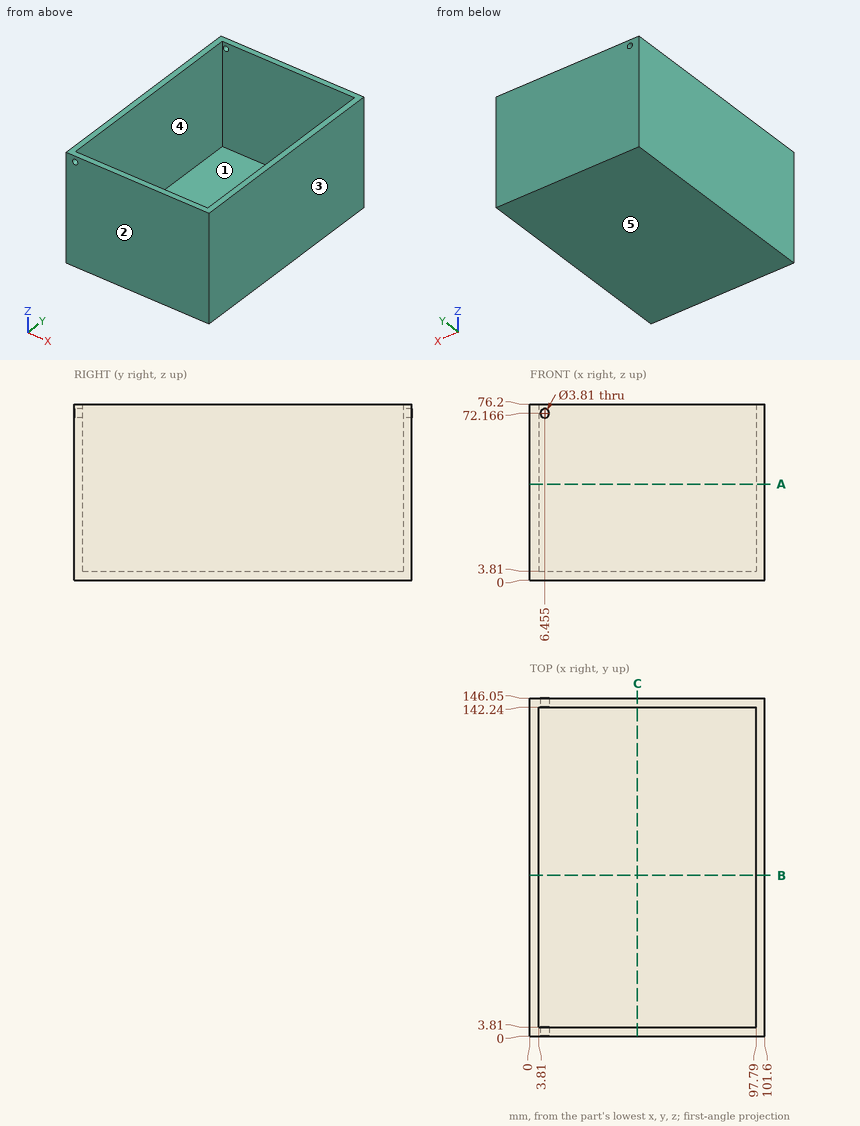
Can you work these out from the drawing? Everything is in mm from the part's minimum corner. A direction names the side the tool comes from. Round coordinates to 2 decimals unless told otherwise and drop trailing zeros. Order: outer loops, then holes, each group sorted by start corner. A loop starts at its lowest first (then second) coordinate and runs counter-clockwise, first axis right, second up. Notation, with made-up numbers: (42, -18) -> (50, -18) arc R12 ccw to (50, 0) -> close; hole circle Ø1 at (33, -28). An arc over 180 degrees is marked (long way). Return JSON: item names as keys, results as strings. Group by question number.
1. We'd pull the mould along Y, two halves only. Please class the marked faces 1, 2 and 3: released by +Y, released by -Y, zero draft, split by the parting line, or undercut.
2. I need wall thicknesses on line 1 (Y direction, x = 49.5, z = 57.5); line 2 (X direction, y = 119, z = 46.5); line 3 (Z direction, x = 14.5, y = 133). Which ranges of each line are inside material? Lowest first, please. Write a range as [from, to].
3. If we section it at C-C, the plane x = 46.5: Write out the boundary of the cut face in (y, z).
4. Will these pins go through, and if not, where does the flat tip stop? pin 1 (10 mm diameter, centred on x = 47.5, y = 106, fed in from +Z); pin 2 (3 mm diameter, centred on x = 6.46, z = 72.17, fed in from +Y).
5. Which directions (+Z, -Z, +X, -X, +Y, -Y) give clear straight access to the entire face, cutting with the end or side of a thin tool? Please do the marked faces 4 and 5.
6. If we section it at B-B, the plane y = 69.5: Write out the boundary of the cut face in (x, z).
7. If we section it at A-A, the plane z = 41.5: Write out the boundary of the cut face in (x, y).
Output values:
{
 "1": {"face 1": "undercut", "face 2": "released by -Y", "face 3": "zero draft"},
 "2": {"line 1": "[0, 3.81], [142.24, 146.05]", "line 2": "[0, 3.81], [97.79, 101.6]", "line 3": "[0, 3.81]"},
 "3": {"outline": "(0, 0) -> (146.05, 0) -> (146.05, 76.2) -> (142.24, 76.2) -> (142.24, 3.81) -> (3.81, 3.81) -> (3.81, 76.2) -> (0, 76.2) -> close"},
 "4": {"pin 1": "z = 3.81", "pin 2": "through"},
 "5": {"face 4": "+Z", "face 5": "-Z, +X, -X, +Y, -Y"},
 "6": {"outline": "(0, 0) -> (101.6, 0) -> (101.6, 76.2) -> (97.79, 76.2) -> (97.79, 3.81) -> (3.81, 3.81) -> (3.81, 76.2) -> (0, 76.2) -> close"},
 "7": {"outline": "(0, 0) -> (101.6, 0) -> (101.6, 146.05) -> (0, 146.05) -> close; hole (3.81, 3.81) -> (97.79, 3.81) -> (97.79, 142.24) -> (3.81, 142.24) -> close"}
}
